Could you check a few things on this drawing? It's one solid part, dimensions in mm from its lowest x, y, z. A direction names the side the tool comes from. Coordinates: 2 decimals unless noted, no trailing zeros. Order: outer loops, then holes, each group sorted by start corner. A loop starts at its lowest first (then second) coordinate and runs counter-clockwise, first axis right, second up. Notation, with made-up numbers: (58, 13.25) -> (85, 13.25) arc R22 cw to (85, 40.25) -> close; hole circle Ø3 at (-16, -13). An arc over 180 degrees is marked (long way). Use a Markdown table: item, result. Add a question column.
1. For the marked faces 1, 2 and 3, which set-ups out of +Z, -Z, +X, -X, +Y, -Y let a thin tool reach every point of the face, with its end or its side?
2. Suppose I cut it at B-B, the plane x = 5.6. List the corners of the cut face in (y, z) for me.
3. Suppose I cut it at A-A, the plane y = 9.5. List the corners of the cut face in (x, z) for me, then the cut area to 3 significant figures.
4. Suppose I cut it at D-D, the plane z = 75.4. List the corners of the cut face in (x, y) for me, then the cut area to 3 significant figures.
5. Suppose I cut it at C-C, the plane z = 22.4. List the corners of the cut face in (x, y) for me, then the cut area to 3 significant figures.
6. If I drill on line 1 along X through (y, z) = (0.9, 75.4); line 2 along Z through (x, y) = (5.6, 0.55); line 3 along X through (y, z) = (1.2, 22.4), over which ranges is the centre line in solid material (lowest first)? Write a range as from..to.
7. For pin 1 Ø24.5 at (x, z) = (46.5, 23) entering from +Y; pin 2 Ø1.5 at (y, z) = (4, 44) entering from -X; pin 3 Ø5 at (x, y) = (104.5, 5) entering from -Z, each with a flat end and sliding along its axis, tell me the tip position at first contact or that it passes through.
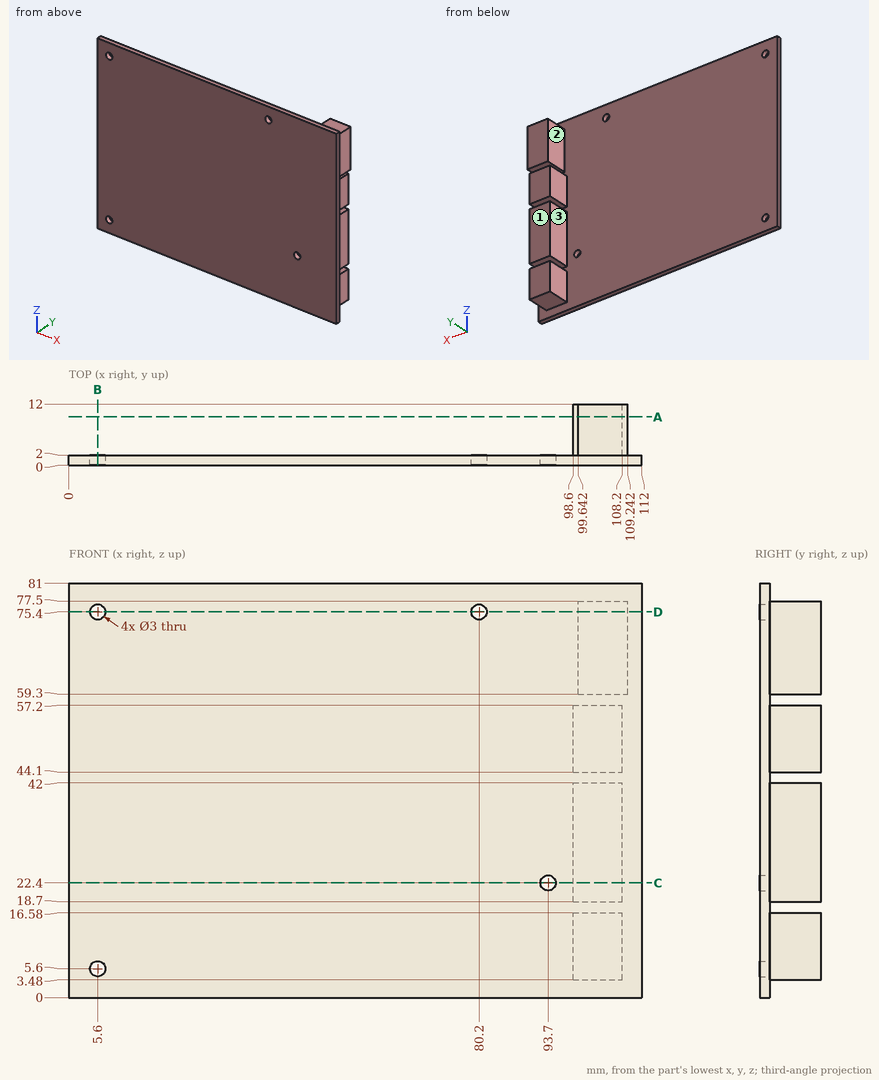
Worked out:
| question | item | result |
|---|---|---|
| 1 | face 1 | +Z, -Z, +X, -X, +Y |
| 1 | face 2 | +Z, -X, +Y |
| 1 | face 3 | +Z, -Z, -X, +Y |
| 2 | outline | (0, 0) -> (2, 0) -> (2, 4.1) -> (0, 4.1) -> close; (0, 7.1) -> (2, 7.1) -> (2, 73.9) -> (0, 73.9) -> close; (0, 76.9) -> (2, 76.9) -> (2, 81) -> (0, 81) -> close |
| 3 | outline | (98.6, 3.48) -> (108.2, 3.48) -> (108.2, 16.58) -> (98.6, 16.58) -> close; (98.6, 18.7) -> (108.2, 18.7) -> (108.2, 42) -> (98.6, 42) -> close; (98.6, 44.1) -> (108.2, 44.1) -> (108.2, 57.2) -> (98.6, 57.2) -> close; (99.64, 59.3) -> (109.24, 59.3) -> (109.24, 77.5) -> (99.64, 77.5) -> close |
| 3 | area | 650 mm² |
| 4 | outline | (0, 0) -> (4.1, 0) -> (4.1, 2) -> (0, 2) -> close; (7.1, 0) -> (78.7, 0) -> (78.7, 2) -> (7.1, 2) -> close; (81.7, 0) -> (112, 0) -> (112, 2) -> (109.24, 2) -> (109.24, 12) -> (99.64, 12) -> (99.64, 2) -> (81.7, 2) -> close |
| 4 | area | 308 mm² |
| 5 | outline | (0, 0) -> (92.2, 0) -> (92.2, 2) -> (0, 2) -> close; (95.2, 0) -> (112, 0) -> (112, 2) -> (108.2, 2) -> (108.2, 12) -> (98.6, 12) -> (98.6, 2) -> (95.2, 2) -> close |
| 5 | area | 314 mm² |
| 6 | line 1 | x = 0..4.1, 7.1..78.7, 81.7..112 |
| 6 | line 2 | z = 0..4.1, 7.1..73.9, 76.9..81 |
| 6 | line 3 | x = 0..92.2, 95.2..112 |
| 7 | pin 1 | stops at y = 2 |
| 7 | pin 2 | stops at x = 98.6 |
| 7 | pin 3 | stops at z = 3.48 |
